Design review of the part built by this model. Coordinates are the model's own, in mm. A direction names the side the tool comes from. Coordinates: 2 decimals unless noted, no trailing zeros. Write each loop counter-clockwise with the first axis right and the second up, starting at its lowest first coordinate (ties: lowest second). Pieces come first, ordered by that corner, then holes. Notation, with made-up numbers: (16, -21) - (52, -21) arc R13 cw to (52, -4) - close; hole circle Ø6 at (85.5, 10). An arc over 180 degrees is marked (long way). Answer as CSV lines item,"result". Start each with the question number.
Q1. We need section D-D (z = -2). Write out the cut boundary in (x, y).
Q2. For line 1 along Z through (x, y) = (-4.5, -0.75); line 2 along X through (y, z) = (-0.65, -0.5); line 3 along X through (y, z) = (0.15, 1.75), list the stretches that pass through material, from the lowest coordinate up. Write a range as [from, to].
Q3. We need section A-A (z = 0). Write out the cut boundary in (x, y), plus the area to 3 significant figures.
Q4. We need section C-C (x = -1.75). Write out the cut boundary in (y, z), plus the area to 3 significant figures.
Q5. We need section B-B (x = 4.5). Write out the cut boundary in (y, z), plus the area to 3 significant figures.
Q6. Clearance check with flat-ended pins moving along their axes: pin 1 (0.5 mm diameter, centred on x = -0.5, y = 0.5, fed in from -Z); pin 2 (3 mm diameter, centred on x = 4.5, z = 0, fed in from -Y); pin 3 (1.8 mm diameter, centred on x = -4.5, z = 0, fed in from -Y) (1 decimal); pin 4 (0.8 mm diameter, centred on y = 0.5, z = 0, fed in from +X). State where each tip first meets the part, or that it passes through.
Q7. Mouldability with a two-part tool opening along X and no side actions: class faces 3 (the face through (0, 0.5, 2.5)), 4 (the face through (-2.5, 0.5, 0)), 5 (the face through (2.5, 0.5, 0)), 6 (the face through (3.5, -0.5, 0)) as pulls with the +X half, pulls with the -X half, needs draft (parallel to the pull), parting line crosses it, or undercut.
Q8. Machinability: for faces 1 (the face through (0, 0.5, -2.5)), 2 (the face through (0, 1, 0)), which of the approach directions +Z, -Z, +X, -X, +Y, -Y give a long, thin tool a straight path to every point of the face, cutting with its end or side? Answer none if there is none.
from build123d import *

# Parameters (mm, degrees)
ESQUISSE1_W        = 5
ESQUISSE1_H        = 5
BOSS_EXTRU_1_DEPTH = 1
ESQUISSE2_W        = 13
ESQUISSE2_H        = 7
ESQUISSE2_R        = 1
BOSS_EXTRU_2_DEPTH = 1


with BuildPart() as part:
    # Esquisse1 → Boss.-Extru.1 (new body)
    with BuildSketch(Plane(origin=(0, 0, 0), x_dir=(1, 0, 0), z_dir=(0, 1, 0))):
        Rectangle(ESQUISSE1_W, ESQUISSE1_H)
    extrude(amount=BOSS_EXTRU_1_DEPTH)

    # Esquisse2 → Boss.-Extru.2 (add)
    with BuildSketch(Plane.XZ):
        Rectangle(ESQUISSE2_W, ESQUISSE2_H)
        with Locations((4.5, 0)):
            Circle(ESQUISSE2_R, mode=Mode.SUBTRACT)
        with Locations((-4.5, 0)):
            Circle(ESQUISSE2_R, mode=Mode.SUBTRACT)
    extrude(amount=BOSS_EXTRU_2_DEPTH)


solid = part.part
Results list:
1,outline,"(-6.5, -1) - (6.5, -1) - (6.5, 0) - (2.5, 0) - (2.5, 1) - (-2.5, 1) - (-2.5, 0) - (-6.5, 0) - close"
2,line 1,"z = [-3.5, -1], [1, 3.5]"
2,line 2,"x = [-6.5, -5.37], [-3.63, 3.63], [5.37, 6.5]"
2,line 3,"x = [-2.5, 2.5]"
3,outline,"(-6.5, -1) - (-5.5, -1) - (-5.5, 0) - (-6.5, 0) - close; (-3.5, -1) - (3.5, -1) - (3.5, 0) - (2.5, 0) - (2.5, 1) - (-2.5, 1) - (-2.5, 0) - (-3.5, 0) - close; (5.5, -1) - (6.5, -1) - (6.5, 0) - (5.5, 0) - close"
3,area,"14.0 mm2"
4,outline,"(-1, -3.5) - (0, -3.5) - (0, -2.5) - (1, -2.5) - (1, 2.5) - (0, 2.5) - (0, 3.5) - (-1, 3.5) - close"
4,area,"12.0 mm2"
5,outline,"(-1, -3.5) - (0, -3.5) - (0, -1) - (-1, -1) - close; (-1, 1) - (0, 1) - (0, 3.5) - (-1, 3.5) - close"
5,area,"5.00 mm2"
6,pin 1,"stops at z = -2.5"
6,pin 2,"stops at y = -1"
6,pin 3,"passes through"
6,pin 4,"stops at x = 2.5"
7,face 3,"needs draft"
7,face 4,"pulls with the -X half"
7,face 5,"pulls with the +X half"
7,face 6,"undercut"
8,face 1,"-Z, +X, -X, +Y"
8,face 2,"+Z, -Z, +X, -X, +Y"
